```python
from build123d import *

# Parameters (mm, degrees)
SKETCH1_R                = 27.5
BOSS_EXTRUDE1_DEPTH      = 15
CHAMFER1_SIZE            = 2
SKETCH2_R                = 17.5
CUT_EXTRUDE1_DEPTH       = 12
SKETCH3_R                = 20.25
CUT_EXTRUDE2_DEPTH       = 3
SKETCH4_R                = 2
CUT_EXTRUDE3_DEPTH       = 42.683330001
BOSS_EXTRUDE2_DEPTH      = 9
SKETCH6_R                = 1.5
CUT_EXTRUDE4_DEPTH       = 41.700123015
CHAMFER2_SIZE            = 2
CHAMFER2_OF_MIRROR1_SIZE = 2
BOSS_EXTRUDE8_START      = 3
BOSS_EXTRUDE8_DEPTH      = 3
SKETCH14_W               = 23
SKETCH14_H               = 12
CUT_EXTRUDE5_DEPTH       = 10
SKETCH16_R               = 1.5
CUT_EXTRUDE6_DEPTH       = 10
SKETCH17_R               = 2.5
CUT_EXTRUDE7_DEPTH       = 6
SKETCH18_R               = 0.875
CUT_EXTRUDE8_DEPTH       = 3
CHAMFER3_SIZE            = 0.8
SKETCH19_W               = 4
SKETCH19_H               = 0.5
BOSS_EXTRUDE9_DEPTH      = 0.5
CHAMFER4_SIZE            = 0.5
LPATTERN1_START          = -8.942375138
LPATTERN1_OUTLINE_W      = 6
LPATTERN1_OUTLINE_H      = 2.185015825
LPATTERN1_DEPTH          = 0.353553391
LPATTERN1_START_2        = -9.649481919
LPATTERN1_2_OUTLINE_W    = 6
LPATTERN1_2_OUTLINE_H    = 0.353553391
LPATTERN1_2_DEPTH        = 0.353553391
LPATTERN1_START_3        = -10.003035309
LPATTERN1_3_OUTLINE_W    = 6
LPATTERN1_3_OUTLINE_H    = 0.353553391
LPATTERN1_3_DEPTH        = 0.35355339
LPATTERN1_START_4        = -9.295928528
LPATTERN1_4_OUTLINE_W    = 6
LPATTERN1_4_OUTLINE_H    = 0.35355339
LPATTERN1_4_DEPTH        = 0.35355339


# Read off the part's stored shape, not the designer's step: LPattern1
with BuildPart() as part:
    # Sketch1 → Boss-Extrude1 (new body)
    with BuildSketch(Plane.XY):
        Circle(SKETCH1_R)
    extrude(amount=BOSS_EXTRUDE1_DEPTH)

    # Chamfer1
    chamfer1_edges = [part.edges().sort_by_distance(p)[0] for p in [
        (-27.5, 0, 15),
    ]]
    chamfer(chamfer1_edges, length=CHAMFER1_SIZE)

    # Sketch2 → Cut-Extrude1 (cut)
    with BuildSketch(Plane.XY.offset(15)):
        Circle(SKETCH2_R)
    extrude(amount=-CUT_EXTRUDE1_DEPTH, mode=Mode.SUBTRACT)

    # Sketch3 → Cut-Extrude2 (cut)
    with BuildSketch(Plane.XY.offset(15)):
        Circle(SKETCH3_R)
    extrude(amount=-CUT_EXTRUDE2_DEPTH, mode=Mode.SUBTRACT)

    # Sketch4 → Cut-Extrude3 (cut, through all)
    with BuildSketch(Plane(origin=(0, 0, 0), x_dir=(1, 0, 0), z_dir=(0, 1, 0))):
        with Locations(Location((0, -5, 0), (0, 0, 270))):
            Circle(SKETCH4_R)
    extrude(amount=-CUT_EXTRUDE3_DEPTH, mode=Mode.SUBTRACT)

    # Sketch5 → Boss-Extrude2 (add)
    with BuildSketch(Plane.XY.offset(12)):
        with BuildLine():
            ThreePointArc((-15.781356255, -1.926213803), (-14.875, 0), (-15.781356255, 1.926213803))
            ThreePointArc((-15.781356255, 1.926213803), (-16.724757779, 3.318673761), (-16.770509831, 5))
            ThreePointArc((-16.770509831, 5), (-17.5, 0), (-16.770509831, -5))
            ThreePointArc((-16.770509831, -5), (-16.724757779, -3.318673761), (-15.781356255, -1.926213803))
        make_face()
    boss_extrude2 = extrude(amount=-BOSS_EXTRUDE2_DEPTH)

    # Sketch6 → Cut-Extrude4 (cut, through all)
    with BuildSketch(Plane.XY.offset(12)):
        with Locations((-17.375, 0)):
            Circle(SKETCH6_R)
    cut_extrude4 = extrude(amount=-CUT_EXTRUDE4_DEPTH, mode=Mode.SUBTRACT)

    # Chamfer2
    chamfer2_edges = [part.edges().sort_by_distance(p)[0] for p in [
        (-18.875, 0, 0),
    ]]
    chamfer(chamfer2_edges, length=CHAMFER2_SIZE)

    # Mirror1: Boss-Extrude2, Cut-Extrude4 across plane
    add(boss_extrude2.mirror(Plane(origin=(0, 0, 0), x_dir=(0, 0, 1), z_dir=(1, 0, 0))))
    add(cut_extrude4.mirror(Plane(origin=(0, 0, 0), x_dir=(0, 0, 1), z_dir=(1, 0, 0))), mode=Mode.SUBTRACT)

    # Chamfer2 of Mirror1
    chamfer2_of_mirror1_edges = [part.edges().sort_by_distance(p)[0] for p in [
        (18.875, 0, 0),
    ]]
    chamfer(chamfer2_of_mirror1_edges, length=CHAMFER2_OF_MIRROR1_SIZE)

    # Sketch8 → Boss-Extrude8 (add)
    with BuildSketch(Plane.XY.offset(3).offset(BOSS_EXTRUDE8_START)):
        with BuildLine():
            Line((-2, -17.385338651), (-2, -14.646428199))
            ThreePointArc((-2, -14.646428199), (-3.5, -13.146428199), (-5, -14.646428199))
            Line((-5, -14.646428199), (-5, -16.770509831))
            ThreePointArc((-5, -16.770509831), (-3.513474579, -17.143672196), (-2, -17.385338651))
        make_face()
    boss_extrude8 = extrude(amount=-BOSS_EXTRUDE8_DEPTH)

    # Sketch14 → Cut-Extrude5 (cut)
    with BuildSketch(Plane.XY.offset(12)):
        with Locations((0, 10.667708301)):
            Rectangle(SKETCH14_W, SKETCH14_H)
    extrude(amount=-CUT_EXTRUDE5_DEPTH, mode=Mode.SUBTRACT)

    # Sketch16 → Cut-Extrude6 (cut, symmetric)
    with BuildSketch(Plane(origin=(14.318912319, -14.318912319, 3), x_dir=(0, 0, -1), z_dir=(0.7071067811865489, -0.7071067811865462, 0))):
        with Locations(Location((-3, 0, 0), (0, 0, 270))):
            Circle(SKETCH16_R)
    cut_extrude6 = extrude(amount=CUT_EXTRUDE6_DEPTH, both=True, mode=Mode.SUBTRACT)

    # Sketch17 → Cut-Extrude7 (cut)
    with BuildSketch(Plane(origin=(12.197591975, -12.197591975, 3), x_dir=(0, 0, -1), z_dir=(0.7071067811865489, -0.7071067811865462, 0))):
        with Locations(Location((-3, 0, 0), (0, 0, 270))):
            Circle(SKETCH17_R)
    cut_extrude7 = extrude(amount=CUT_EXTRUDE7_DEPTH, mode=Mode.SUBTRACT)

    # Mirror2: Cut-Extrude6, Cut-Extrude7 across plane
    add(cut_extrude6.mirror(Plane(origin=(0, 0, 0), x_dir=(0, 0, 1), z_dir=(1, 0, 0))), mode=Mode.SUBTRACT)
    add(cut_extrude7.mirror(Plane(origin=(0, 0, 0), x_dir=(0, 0, 1), z_dir=(1, 0, 0))), mode=Mode.SUBTRACT)

    # Sketch18 → Cut-Extrude8 (cut)
    with BuildSketch(Plane.XY.offset(6)):
        with Locations((-3.5, -14.646428199)):
            Circle(SKETCH18_R)
    cut_extrude8 = extrude(amount=-CUT_EXTRUDE8_DEPTH, mode=Mode.SUBTRACT)

    # Mirror5: Boss-Extrude8, Cut-Extrude8 across plane
    add(boss_extrude8.mirror(Plane(origin=(0, 0, 0), x_dir=(0, 0, 1), z_dir=(1, 0, 0))))
    add(cut_extrude8.mirror(Plane(origin=(0, 0, 0), x_dir=(0, 0, 1), z_dir=(1, 0, 0))), mode=Mode.SUBTRACT)

    # Chamfer3
    chamfer3_edges = [part.edges().sort_by_distance(p)[0] for p in [
        (-4.375, -14.646428199, 3),
        (4.375, -14.646428199, 3),
    ]]
    chamfer(chamfer3_edges, length=CHAMFER3_SIZE)

    # Sketch19 → Boss-Extrude9 (add)
    with BuildSketch(Plane.XY.offset(3)):
        with Locations((0, -14.896428199)):
            Rectangle(SKETCH19_W, SKETCH19_H)
    extrude(amount=BOSS_EXTRUDE9_DEPTH)

    # Chamfer4
    # the kernel refuses this chamfer: 0.5 mm, written as the material it takes off along each edge
    with BuildSketch(Plane(origin=(-2, -15.146428199, 3.5), x_dir=(0, -0.027495876610585623, -0.9996219169112968), z_dir=(1, 0, 0))) as chamfer4_piece_1:
        Polygon((CHAMFER4_SIZE * 0.999621916911, CHAMFER4_SIZE * 0.0274958766106), (-CHAMFER4_SIZE * 0.0274958766106, CHAMFER4_SIZE * 0.999621916911), (0, 0), align=None)
    extrude(amount=4, mode=Mode.SUBTRACT)
    with BuildSketch(Plane(origin=(2, -14.646428199, 3.5), x_dir=(0, -0.9996219169112968, 0.02749587661058651), z_dir=(-1, 0, 0))) as chamfer4_piece_2:
        Polygon((CHAMFER4_SIZE * 0.999621916911, -CHAMFER4_SIZE * 0.0274958766106), (-CHAMFER4_SIZE * 0.0274958766106, -CHAMFER4_SIZE * 0.999621916911), (0, 0), align=None)
    extrude(amount=4, mode=Mode.SUBTRACT)

    # LPattern1 outline → LPattern1 (add)
    with BuildSketch(Plane(origin=(0, 0, 0), x_dir=(1, 0, 0), z_dir=(0, 0.7071067811865476, 0.7071067811865476)).offset(LPATTERN1_START)):
        with Locations((0, -12.092507913)):
            Rectangle(LPATTERN1_OUTLINE_W, LPATTERN1_OUTLINE_H)
    extrude(amount=LPATTERN1_DEPTH)

    # LPattern1 2 outline → LPattern1 2 (add)
    with BuildSketch(Plane(origin=(0, 0, 0), x_dir=(1, 0, 0), z_dir=(0, 0.7071067811865476, 0.7071067811865476)).offset(LPATTERN1_START_2)):
        with Locations((0, -13.715345911)):
            Rectangle(LPATTERN1_2_OUTLINE_W, LPATTERN1_2_OUTLINE_H)
    extrude(amount=LPATTERN1_2_DEPTH)

    # LPattern1 3 outline → LPattern1 3 (add)
    with BuildSketch(Plane(origin=(0, 0, 0), x_dir=(1, 0, 0), z_dir=(0, 0.7071067811865476, 0.7071067811865476)).offset(LPATTERN1_START_3)):
        with Locations((0, -14.068899302)):
            Rectangle(LPATTERN1_3_OUTLINE_W, LPATTERN1_3_OUTLINE_H)
    extrude(amount=LPATTERN1_3_DEPTH)

    # LPattern1 4 outline → LPattern1 4 (add)
    with BuildSketch(Plane(origin=(0, 0, 0), x_dir=(1, 0, 0), z_dir=(0, 0.7071067811865476, 0.7071067811865476)).offset(LPATTERN1_START_4)):
        with Locations((0, -13.36179252)):
            Rectangle(LPATTERN1_4_OUTLINE_W, LPATTERN1_4_OUTLINE_H)
    extrude(amount=LPATTERN1_4_DEPTH)


solid = part.part
```
Part model, mm, in its own coordinate system. A direction names the side the tool comes from. Coordinates: 2 decimals unless noted, no trailing zeros. Write each loop counter-clockwise with the first axis right and the second up, starting at its lowest first coordinate (ties: lowest second). Pieces come first, ordered by that corner, then holes.
Item 1: Which spindle directions (+Z, -Z, +X, -X, +Y, -Y) get a long thin tool onto all of the face, cutting with end or side? Do faces 4 (the face through (-18.874, 0.066, 7.07)), 5 (the face through (-14.679, 9.528, 7.563)). Say none if no direction does.
Item 2: Slice it at A-A (y = 0). Write the cut outline in (x, z) (3 decimals).
Item 3: Mould opens along X. For faces 1 (the face through (3.307, -14.586, 3.128)), 2 (the face through (7.44, 19.01, 15)), 3 (the face through (-5.961, -26.846, 6.409)) say: released by +X, released by -X, zero draft, split by the parting line, or undercut.
Item 4: Pin check, flat tips, straight feed: pin 1 (1 mm diameter, centred on x = 15, y = 1, fed in from -Z); pin 2 (18.5 mm diameter, centred on x = 8.5, y = 4, fed in from +Z); pin 3 (5 mm diameter, centred on x = 5, z = 2, fed in from -Y). Stop position of each tip, or through.
Item 5: Probe line 1 (Y direction, x = 0, z = 12.9); line 2 (Z direction, x = 0, y = -22.5); line 3 (Y direction, x = 14.5, z = 5.25). List the from-to ranges inside material, lowest first.
Results found:
1. face 4: +Z, -Z
1. face 5: +Z
2. outline: (-27.5, 0) - (-20.875, 0) - (-18.875, 2) - (-18.875, 12) - (-20.25, 12) - (-20.25, 15) - (-25.5, 15) - (-27.5, 13) - close; (-15.875, 2) - (-13.875, 0) - (13.875, 0) - (15.875, 2) - (15.875, 12) - (14.875, 12) - (14.875, 3) - (-14.875, 3) - (-14.875, 12) - (-15.875, 12) - close; (18.875, 2) - (20.875, 0) - (27.5, 0) - (27.5, 13) - (25.5, 15) - (20.25, 15) - (20.25, 12) - (18.875, 12) - close
3. face 1: undercut
3. face 2: zero draft
3. face 3: split by the parting line
4. pin 1: stops at z = 0.42
4. pin 2: stops at z = 12
4. pin 3: stops at y = -27.39
5. line 1: y = -27.5 to -20.25, 20.25 to 27.5
5. line 2: z = 0 to 3, 7 to 15
5. line 3: y = -23.37 to -17.87, -11.13 to -9.8, 9.8 to 23.37
